For this review, take the finished solid that the model builds, in its own axes (mm). Coordinates: 2 decimals unless noted, no trailing zeros. Write each loop counter-clockwise with the first axis right and the second up, starting at its lowest first coordinate (ties: lowest second). Pieces come first, ordered by that corner, then holes.
1) To check wall thickness, follow line 1 along Z through (x, y) = (49, -1.5); line 2 along Z through (x, y) = (45.5, -1.6); line 3 along X through (y, z) = (-2.5, -30.2). State the ranges of each line that lie inside material, in increasing order.
2) We need section A-A on y = -2.7. Write out the cut boundary in (x, z).
3) We need section B-B on x = 0. Write out the cut boundary in (y, z), then the cut area to 3 significant figures.
4) We need section D-D on z = -16.5. Write out the cut boundary in (x, y), then the cut area to 3 significant figures.
5) Mouldability with a two-part tool opening along X and no side actions: class faces 1 (the face through (46, -2, -27.95)), 2 (the face through (49.744, -1.972, -30.298)), 3 (the face through (1.29, -2.03, -2.9)) as pulls with the +X half, pulls with the -X half, needs draft (parallel to the pull), parting line crosses it, or undercut.
6) We need section C-C on z = 0. Write out the cut boundary in (x, y).
7) Insertion check: P1, Ø1.4, axis at x = 0, z = 0, coming from the +Y side; P2, Ø2, axis at x = 40, y = -0.5, coming from the +Z side; P3, Ø1, axis at y = -1.5, z = -25.5, coming from the -X side; P4, Ø1, axis at y = -3.5, z = -3, coming from the +X side. Each pin has a flat end and moves straight along its axis. Give the tip position at first contact, or say it passes through.
from build123d import *

# Parameters (mm, degrees)
SKETCH1_R           = 0.75
BOSS_EXTRUDE1_DEPTH = 4
FILLET1_R           = 10


with BuildPart() as part:
    # Sketch1 → Boss-Extrude1 (new body)
    with BuildSketch(Plane(origin=(0, 0, 0), x_dir=(1, 0, 0), z_dir=(0, 1, 0))):
        with BuildLine():
            Line((49, 32.45), (39, 32.45))
            Line((39, 32.45), (0.6574204, 2.151812821))
            ThreePointArc((0.6574204, 2.151812821), (-2.211145355, -0.416336667), (1.394986025, -1.765365115))
            Line((1.394986025, -1.765365115), (39, 27.95))
            Line((39, 27.95), (49, 27.95))
            ThreePointArc((49, 27.95), (51.25, 30.2), (49, 32.45))
        make_face()
        with Locations(Location((49, 30.2, 0), (0, 0, 270))):
            Circle(SKETCH1_R, mode=Mode.SUBTRACT)
        with Locations(Location((0, 0, 0), (0, 0, 270))):
            Circle(SKETCH1_R, mode=Mode.SUBTRACT)
    extrude(amount=-BOSS_EXTRUDE1_DEPTH)

    # Fillet1
    fillet1_edges = [part.edges().sort_by_distance(p)[0] for p in [
        (39, -2, -27.95),
        (0.6574204, -2, -2.151812821),
        (39, -2, -32.45),
    ]]
    fillet(fillet1_edges, radius=FILLET1_R)


solid = part.part
Result:
1. line 1: z = -32.45 to -30.95, -29.45 to -27.95
1. line 2: z = -32.45 to -27.95
1. line 3: x = 36.15 to 48.25, 49.75 to 51.25
2. outline: (-0.6, -2.17) arc R10 cw to (2.95, -3.97) - (36.27, -30.3) arc R10 ccw to (42.47, -32.45) - (49, -32.45) arc R2.25 ccw to (49, -27.95) - (42.47, -27.95) arc R10 cw to (36.27, -25.8) - (1.39, 1.77) arc R2.25 ccw (long way) to start; hole circle Ø1.5 at (0, 0); hole circle Ø1.5 at (49, -30.2)
3. outline: (-4, -2.35) - (0, -2.35) - (0, -0.75) - (-4, -0.75) - close; (-4, 0.75) - (0, 0.75) - (0, 2.25) - (-4, 2.25) - close
3. area: 12.4 mm2
4. outline: (18.82, -4) - (24.51, -4) - (24.51, 0) - (18.82, 0) - close
4. area: 22.8 mm2
5. face 1: needs draft
5. face 2: undercut
5. face 3: pulls with the -X half
6. outline: (-2.25, -4) - (-0.75, -4) - (-0.75, 0) - (-2.25, 0) - close; (0.75, -4) - (3.63, -4) - (3.63, 0) - (0.75, 0) - close
7. P1: passes through
7. P2: stops at z = -27.33
7. P3: stops at x = 29.57
7. P4: stops at x = 8.06
